Read the model definition and answer for the solid it produces. Units are mm, in the model's axes. Coordinates: 2 decimals unless noted, no trailing zeros. Write each loop counter-clockwise with the first axis right and the second up, starting at its lowest first coordinate (ties: lowest second). Pieces come first, ordered by that corner, then holes.
(1) Section C-C on y = 12.25 is taken. Write down the section's boundary in (x, z), then the cut area to 3 significant figures.
(2) Find the intervals of material crossed by probe 1 along Y at (x, z) = (40, 7); probe 2 along X at (y, z) = (9.75, 4.25); probe 3 along X at (y, z) = (9.25, 10), in increasing order.
(3) Given pin 1 (1.5 mm diameter, centred on x = 30, y = 8, fed in from -Z); pin 2 (3 mm diameter, centred on y = 1.5, z = 8.5, fed in from -X), each flat-ended and moving along its own axis, determine where each tip first touches the part or whether it passes through.
(4) The mould has two halves that part along Y. Classify faces 1 (the cylindrical face through (2, 7.6, 4.9)), 2 (the cylindrical face through (43, 14, 6)), 3 (the flat face through (45, 7, 5)), 4 (the cylindrical face through (37, 7.6, 4.9)): +Y half, -Y half, draft (parallel to the pull), parting line (faces both ways), or undercut.
(5) Section A-A on y = 7.5 is taken. Write down the section's boundary in (x, z), then the cut area to 3 significant figures.
(6) Section B-B on z = 1.5 is taken. Write down the section's boundary in (x, y), then the cut area to 3 significant figures.
from build123d import *

# Parameters (mm, degrees)
CROQUIS1_W              = 45
CROQUIS1_H              = 15
CROQUIS1_R              = 3
SALIENTE_EXTRUIR1_DEPTH = 11
REDONDEO1_R             = 5
CHAFL_N1_SIZE           = 1


with BuildPart() as part:
    # Croquis1 → Saliente-Extruir1 (new body)
    with BuildSketch(Plane.XY):
        with Locations((22.5, 7.5)):
            Rectangle(CROQUIS1_W, CROQUIS1_H)
        with Locations((5, 7.5)):
            Circle(CROQUIS1_R, mode=Mode.SUBTRACT)
        with Locations((40, 7.5)):
            Circle(CROQUIS1_R, mode=Mode.SUBTRACT)
    extrude(amount=SALIENTE_EXTRUIR1_DEPTH)

    # Redondeo1
    redondeo1_edges = [part.edges().sort_by_distance(p)[0] for p in [
        (0, 0, 5.5),
        (0, 15, 5.5),
        (45, 15, 5.5),
        (45, 0, 5.5),
    ]]
    fillet(redondeo1_edges, radius=REDONDEO1_R)

    # Chaflán1
    chafl_n1_edges = [part.edges().sort_by_distance(p)[0] for p in [
        (2, 7.5, 11),
        (37, 7.5, 11),
    ]]
    chamfer(chafl_n1_edges, length=CHAFL_N1_SIZE)


solid = part.part
Response:
1. outline: (0.53, 0) - (44.47, 0) - (44.47, 11) - (0.53, 11) - close
1. area: 483 mm2
2. probe 1: y = 0 to 4.5, 10.5 to 15
2. probe 2: x = 0 to 3.02, 6.98 to 38.02, 41.98 to 45
2. probe 3: x = 0 to 2.56, 7.44 to 37.56, 42.44 to 45
3. pin 1: stops at z = 0
3. pin 2: stops at x = 0.42
4. face 1: undercut
4. face 2: +Y half
4. face 3: draft
4. face 4: undercut
5. outline: (0, 0) - (2, 0) - (2, 10) - (1, 11) - (0, 11) - close; (8, 0) - (37, 0) - (37, 10) - (36, 11) - (9, 11) - (8, 10) - close; (43, 0) - (45, 0) - (45, 11) - (44, 11) - (43, 10) - close
5. area: 361 mm2
6. outline: (0, 5) arc R5 ccw to (5, 0) - (40, 0) arc R5 ccw to (45, 5) - (45, 10) arc R5 ccw to (40, 15) - (5, 15) arc R5 ccw to (0, 10) - close; hole circle Ø6 at (5, 7.5); hole circle Ø6 at (40, 7.5)
6. area: 597 mm2
